Verification items for the finished model (mm, model axes). Face numbers are marked on the shaded views. A direction names the side the tool comes from. Give positions to 0.01 mm unless a question says otherwise; leave off trailing zeros. Order: outer loops, then holes, each group sorted by start corner. A loop starts at its lowest first (then second) coordinate and runs counter-clockwise, first axis right, second up.
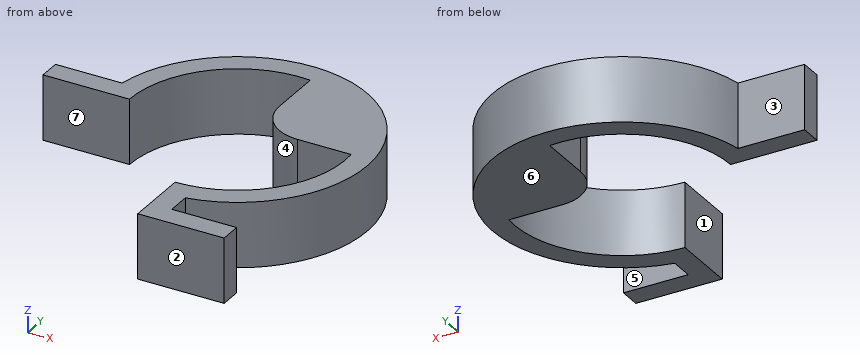
from build123d import *

# Parameters (mm, degrees)
F1_DEPTH = 9.525


with BuildPart() as f1:
    # F0 (on Top) → F1 (new body)
    with BuildSketch(Plane.XY):
        with BuildLine():
            ThreePointArc((15.795426, 1.5875), (11.773215, -10.649274), (0, -15.875))
            Line((0, -15.875), (0, -25.4))
            Line((0, -25.4), (12.7, -25.4))
            Line((12.7, -25.4), (12.7, -22.225))
            Line((12.7, -22.225), (3.175, -22.225))
            Line((3.175, -22.225), (3.175, -18.783553))
            ThreePointArc((3.175, -18.783553), (13.470384, 13.470384), (-18.783553, 3.175))
            Line((-18.783553, 3.175), (-28.575, 3.175))
            Line((-28.575, 3.175), (-28.575, 0))
            Line((-28.575, 0), (-15.875, 0))
            ThreePointArc((-15.875, 0), (-10.649274, 11.773215), (1.5875, 15.795426))
            Line((1.5875, 15.795426), (1.5875, 7.9375))
            ThreePointArc((1.5875, 7.9375), (3.447372, 3.447372), (7.9375, 1.5875))
            Line((7.9375, 1.5875), (15.795426, 1.5875))
        make_face()
    extrude(amount=F1_DEPTH)


solid = f1.part
(1) Release check for a two-part mould opening along Y. For the marked faces 5, 6 and 7 record: pulls with the +Y half, pulls with the -Y half, needs draft (parallel to the pull), parting line crosses it, or undercut.
Solved:
face 5: undercut
face 6: needs draft
face 7: pulls with the -Y half
(2) Section check B-B, the plane y = 10.5. Enter the section's corners in (x, z) (1 decimal), then the cut area to 3 significant figures.
Solved:
outline: (-15.9, 0) - (-11.9, 0) - (-11.9, 9.5) - (-15.9, 9.5) - close; (1.6, 0) - (15.9, 0) - (15.9, 9.5) - (1.6, 9.5) - close
area: 174 mm2
(3) Set-up check for the marked faces 1, 2, 3 and 4: record each of +Z, -Z, +X, -X, +Y, -Y from which the full face is reachable in a straight line by a thin tool's end or side.
Solved:
face 1: +Z, -Z, -X, -Y
face 2: +Z, -Z, +X, -X, -Y
face 3: +Z, -Z, -X, +Y
face 4: +Z, -Z
(4) Section check C-C, the plane x = -10.5. Enter the section's corners in (y, z) (3 decimals).
Solved:
outline: (11.907, 0) - (15.895, 0) - (15.895, 9.525) - (11.907, 9.525) - close
(5) Section check D-D, the plane y = -19.5. Enter the section's corners in (x, z) (3 decimals), then the cut area to 3 significant figures.
Solved:
outline: (0, 0) - (3.175, 0) - (3.175, 9.525) - (0, 9.525) - close
area: 30.2 mm2
(6) Scan lines: line 1 (Y direction, x = 10, z = 6.5) (1 decimal); line 2 (Y direction, x = 10.5, z = 3.5) (1 decimal); line 3 (X direction, y = 0.5, z = 2) (3 decimals). Record each from-to range of solid material in increasing order.
Solved:
line 1: y = -25.4 to -22.2, -16.2 to -12.3, 1.6 to 16.2
line 2: y = -25.4 to -22.2, -15.9 to -11.9, 1.6 to 15.9
line 3: x = -28.575 to -15.867, 15.867 to 19.043
(7) Go/stop test with flat-tipped pins: pin 1 (2 mm diameter, centred on y = -17, z = 1.5, fed in from +X); pin 2 (3.5 mm diameter, centred on y = -24.5, z = 6, fed in from +X); pin 3 (5 mm diameter, centred on x = -10, z = 6, fed in from -Y). Record where each tip stops, or that it passes through.
Solved:
pin 1: stops at x = 10.34
pin 2: stops at x = 12.7
pin 3: stops at y = 9.79
